Can you work these out from the model? Positions are in its coordinate system, mm. Coordinates: 2 decimals unless noted, no trailing zeros. Answer as a JSON object with one key per item and string values. Group by question number.
(1) If we mould it in two halves opening along Z, with no side actions, what happens to faces 1 (the conical face through (4.3, 1.1, -165.7)), 2 (the flat face through (0, 3.175, -3))? For each: pulls with the +Z half, pulls with the -Z half, needs draft (parallel to the pull), parting line crosses it, or undercut.
(2) For pin 1 (4 mm diameter, centred on x = -7.5, z = 113, fed in from -Y); pin 2 (2.5 mm diameter, centred on x = -5, z = 168, fed in from +Y), each with a flat end and sliding along its axis, tell me the tip position at first contact or that it passes through.
(3) I need wall thicknesses on line 1 (X direction, y = 0.45, z = -168); line 2 (X direction, y = 1.85, z = -100); line 3 (Z direction, x = 6.75, y = 2.3). Which ranges of each line are inside material? Lowest first, please.
(4) I want a section at A-A, the plane y = 1.8. State how many separate pieces and enclosed holes the cut face has, plus the area to 3 significant figures.
from build123d import *

# Parameters (mm, degrees)
SKETCH1_W                    = 20
SKETCH1_H                    = 365
BOSS_EXTRUDE1_DEPTH          = 3.175
CSK_FOR_M4_SFHCS1_AT_2_COUNT = 2
CSK_FOR_M4_SFHCS1_AT_2_PITCH = 14.142135624
CSK_FOR_M4_SFHCS1_AT_3_COUNT = 2
CSK_FOR_M4_SFHCS1_AT_3_PITCH = 10
CSK_FOR_M4_SFHCS1_AT_4_COUNT = 2
CSK_FOR_M4_SFHCS1_AT_4_PITCH = 10
CSK_FOR_M4_SFHCS1_AT_5_COUNT = 2
CSK_FOR_M4_SFHCS1_AT_5_PITCH = 346
CSK_FOR_M4_SFHCS1_AT_6_COUNT = 2
CSK_FOR_M4_SFHCS1_AT_6_PITCH = 336.148776586
CSK_FOR_M4_SFHCS1_AT_7_COUNT = 2
CSK_FOR_M4_SFHCS1_AT_7_PITCH = 346.144478506
CSK_FOR_M4_SFHCS1_AT_8_COUNT = 2
CSK_FOR_M4_SFHCS1_AT_8_PITCH = 336
M4X0_7_TAPPED_HOLE1_D        = 3.3


with BuildPart() as part:
    # Sketch1 → Boss-Extrude1 (new body)
    with BuildSketch(Plane(origin=(0, 0, 0), x_dir=(1, 0, 0), z_dir=(0, 1, 0))):
        Rectangle(SKETCH1_W, SKETCH1_H)
    extrude(amount=BOSS_EXTRUDE1_DEPTH)

    # Sketch3 → CSK for M4 SFHCS1 (revolve, cut)
    with BuildSketch(Plane(origin=(5, 3.175, 168), x_dir=(0, 0, 1), z_dir=(1, 0, 0))):
        Polygon((0, 0), (0, 3.175), (2.25, 3.175), (2.25, 2.23), (4.48, 0), align=None)
    csk_for_m4_sfhcs1 = revolve(axis=Axis((5, 9.525, 168), (0, -1, 0)), mode=Mode.SUBTRACT)

    # CSK for M4 SFHCS1 at 2: CSK for M4 SFHCS1 ×2
    with Locations(*[Vector(-0.7071067811865469, 0, 0.7071067811865482) * (i * CSK_FOR_M4_SFHCS1_AT_2_PITCH) for i in range(1, CSK_FOR_M4_SFHCS1_AT_2_COUNT)]):
        add(csk_for_m4_sfhcs1, mode=Mode.SUBTRACT)

    # CSK for M4 SFHCS1 at 3: CSK for M4 SFHCS1 ×2
    with Locations(*[(-i * CSK_FOR_M4_SFHCS1_AT_3_PITCH, 0, 0) for i in range(1, CSK_FOR_M4_SFHCS1_AT_3_COUNT)]):
        add(csk_for_m4_sfhcs1, mode=Mode.SUBTRACT)

    # CSK for M4 SFHCS1 at 4: CSK for M4 SFHCS1 ×2
    with Locations(*[(0, 0, i * CSK_FOR_M4_SFHCS1_AT_4_PITCH) for i in range(1, CSK_FOR_M4_SFHCS1_AT_4_COUNT)]):
        add(csk_for_m4_sfhcs1, mode=Mode.SUBTRACT)

    # CSK for M4 SFHCS1 at 5: CSK for M4 SFHCS1 ×2
    with Locations(*[(0, 0, -i * CSK_FOR_M4_SFHCS1_AT_5_PITCH) for i in range(1, CSK_FOR_M4_SFHCS1_AT_5_COUNT)]):
        add(csk_for_m4_sfhcs1, mode=Mode.SUBTRACT)

    # CSK for M4 SFHCS1 at 6: CSK for M4 SFHCS1 ×2
    with Locations(*[Vector(-0.029748732396333223, 0, -0.9995574085167952) * (i * CSK_FOR_M4_SFHCS1_AT_6_PITCH) for i in range(1, CSK_FOR_M4_SFHCS1_AT_6_COUNT)]):
        add(csk_for_m4_sfhcs1, mode=Mode.SUBTRACT)

    # CSK for M4 SFHCS1 at 7: CSK for M4 SFHCS1 ×2
    with Locations(*[Vector(-0.028889670703889703, 0, -0.9995826063545828) * (i * CSK_FOR_M4_SFHCS1_AT_7_PITCH) for i in range(1, CSK_FOR_M4_SFHCS1_AT_7_COUNT)]):
        add(csk_for_m4_sfhcs1, mode=Mode.SUBTRACT)

    # CSK for M4 SFHCS1 at 8: CSK for M4 SFHCS1 ×2
    with Locations(*[(0, 0, -i * CSK_FOR_M4_SFHCS1_AT_8_PITCH) for i in range(1, CSK_FOR_M4_SFHCS1_AT_8_COUNT)]):
        add(csk_for_m4_sfhcs1, mode=Mode.SUBTRACT)

    # M4x0.7 Tapped Hole1 (through all)
    with Locations(Plane(origin=(0, 3.175, 0), x_dir=(1, 0, 0), z_dir=(0, 1, 0))):
        with Locations((-5, -100), (-5, 100), (5, 100), (5, -100)):
            Hole(M4X0_7_TAPPED_HOLE1_D / 2)


solid = part.part
Computed values:
{
 "1": {"face 1": "undercut", "face 2": "needs draft"},
 "2": {"pin 1": "stops at y = 0", "pin 2": "passes through"},
 "3": {"line 1": "x = -10 to -7.25, -2.75 to 2.75, 7.25 to 10", "line 2": "x = -10 to -6.65, -3.35 to 3.35, 6.65 to 10", "line 3": "z = -182.5 to -181.15, -174.85 to -171.15, -164.85 to 164.85, 171.15 to 174.85, 181.15 to 182.5"},
 "4": {"separate pieces": "1", "enclosed holes": "12", "area": "7,020 mm2"}
}
